from build123d import *

# Parameters (mm, degrees)
SKETCH1_W           = 219.075
SKETCH1_H           = 28.575
BOSS_EXTRUDE1_DEPTH = 12.7
SKETCH2_W           = 211.582
SKETCH2_H           = 22.352
CUT_EXTRUDE1_DEPTH  = 6.35
SKETCH4_R           = 2.794
CUT_EXTRUDE2_DEPTH  = 222.021964406


with BuildPart() as part:
    # Sketch1 → Boss-Extrude1 (new body)
    with BuildSketch(Plane(origin=(0, 0, 0), x_dir=(1, 0, 0), z_dir=(0, 1, 0))):
        with Locations((109.5375, 14.2875)):
            Rectangle(SKETCH1_W, SKETCH1_H)
    extrude(amount=BOSS_EXTRUDE1_DEPTH)

    # Sketch2 → Cut-Extrude1 (cut)
    with BuildSketch(Plane(origin=(0, 12.7, 0), x_dir=(1, 0, 0), z_dir=(0, 1, 0))):
        with Locations((109.5375, 14.2875)):
            Rectangle(SKETCH2_W, SKETCH2_H)
    extrude(amount=-CUT_EXTRUDE1_DEPTH, mode=Mode.SUBTRACT)

    # Sketch4 → Cut-Extrude2 (cut, through all)
    with BuildSketch(Plane(origin=(0, 6.35, 0), x_dir=(1, 0, 0), z_dir=(0, 1, 0))):
        with Locations(Location((11.0363, 19.2405, 0), (0, 0, 270))):
            Circle(SKETCH4_R)
        with Locations(Location((11.0363, 9.3345, 0), (0, 0, 90))):
            Circle(SKETCH4_R)
        with Locations(Location((208.0387, 9.3345, 0), (0, 0, 270))):
            Circle(SKETCH4_R)
        with Locations(Location((208.0387, 19.2405, 0), (0, 0, 90))):
            Circle(SKETCH4_R)
    extrude(amount=-CUT_EXTRUDE2_DEPTH, mode=Mode.SUBTRACT)


solid = part.part
Check sheet for the modelled part. Datum: model origin and axes. Units: mm. A direction names the side the tool comes from. Round coordinates to 2 decimals unless told otherwise and drop trailing zeros. Loops run counter-clockwise (first coordinate to the right, second up) from the corner with the lowest first, then second, coordinate; pieces in that order, holes last.
1. Sectioned sample at C-C on y = 3.5. Record the boundary of the cut face in (x, z) (1 decimal), and give its area (3 significant figures).
2. Set-up check for faces 1 (the flat face through (215.328, 10, -14)), 2 (the flat face through (108, 6, 0)): record each of +Z, -Z, +X, -X, +Y, -Y from which the full face is reachable in a straight line by a thin tool's end or side.
3. Sectioned sample at B-B on z = -18.5. Give the number of separate pieces and of enclosed holes in the cut face, and give its area (3 significant figures).
4. Scan lines: probe 1 along X at (y, z) = (10, -19) (1 decimal); probe 2 along Z at (x, y) = (197.5, 7.25) (1 decimal); probe 3 along X at (y, z) = (1.25, -11.5) (3 decimals). Record each from-to range of solid material in increasing order.
5. Gauge pin test, flat ends, axial feed: pin 1 Ø2 at (x, z) = (91.5, -15.5) entering from -Y; pin 2 Ø6.5 at (x, z) = (11.04, -9.33) entering from +Y; pin 3 Ø5 at (x, z) = (208.04, -19.24) entering from -Y. Record the tip position at first contact, or that the pin passes through.
6. Mould release check, pull along X, two halves, no side actions. Record for faces 3 (the flat face through (3.746, 10, -14)), 4 (the flat face through (0, 6, -14)), 5 (the flat face through (92.8, 12.7, -2.7)): released by +X, released by -X, zero draft, split by the parting line, or undercut.
Recorded:
1. outline: (0, -28.6) - (219.1, -28.6) - (219.1, 0) - (0, 0) - close; hole circle Ø5.6 at (11, -19.2); hole circle Ø5.6 at (11, -9.3); hole circle Ø5.6 at (208, -19.2); hole circle Ø5.6 at (208, -9.3)
1. area: 6,160 mm2
2. face 1: +Y
2. face 2: +Z, +X, -X, +Y, -Y
3. separate pieces: 3
3. enclosed holes: 0
3. area: 1,370 mm2
4. probe 1: x = 0 to 3.7, 215.3 to 219.1
4. probe 2: z = -28.6 to -25.5, -3.1 to 0
4. probe 3: x = 0 to 9.271, 12.802 to 206.273, 209.804 to 219.075
5. pin 1: stops at y = 0
5. pin 2: stops at y = 6.35
5. pin 3: passes through
6. face 3: undercut
6. face 4: released by -X
6. face 5: zero draft
